Here's how the part is built. I have some questions about the finished solid (model axes, mm). Face numbers are marked on the shaded views. A direction names the side the tool comes from. Coordinates: 2 decimals unless noted, no trailing zeros. Write each loop counter-clockwise with the first axis right and the second up, starting at its lowest first coordinate (ties: lowest second). Pieces come first, ordered by that corner, then holes. Notation, with made-up numbers: (-13, 74) -> (16, 74) arc R17 cw to (16, 85) -> close; hole circle Ø3 at (21.5, -11). An arc over 180 degrees is marked (long way). Put each result on its own line as item: value. Start each with the question number.
Item 1: For pin 1 (12 mm diameter, centred on x = 14.5, y = 53, fed in from -Z); pin 2 (4 mm diameter, centred on y = 10, z = 292.5, fed in from +X); pin 3 (4 mm diameter, centred on x = 10, z = 116, fed in from +Y); pin 4 (5 mm diameter, centred on x = 20, z = 262.5, fed in from +Y), each with a flat end and sliding along its axis, tell me the tip position at first contact or that it passes through.
Item 2: I want a section at C-C, the plane x = 45. List the corners of the cut face in (y, z) for me.
Item 3: On a 3-axis mill with a long thin cutter (end or side, diameter ignored), from which of +Z, -Z, +X, -X, +Y, -Y can I reach the whole of each face in a straight line? I mean the marked faces 1 and 2. Say none if no direction works.
Item 4: I want a section at A-A, the plane z = 36. List the corners of the cut face in (x, y) for me.
Item 5: I need wall thicknesses on line 1 (X direction, y = 64, z = 130); line 2 (X direction, y = 4, z = 23). Which ranges of each line are inside material? Lowest first, please. Write a range as [from, to].
Item 6: I want a section at B-B, the plane y = 67.5. List the corners of the cut face in (x, z) for me, then the cut area to 3 significant figures.
Autodesk Inventor part; units mm, degrees
ref_plane "Start plane" through (0, 0, -10.521) normal (0, 0, 1) x (1, 0, 0)
ref_plane "End plane" through (0, 0, 342.7905) normal (0, 0, 1) x (1, 0, 0)
ref_plane "Work Plane3" through (50.8, 38.1, -10.521) normal (-0.3827, 0, -0.9239) x (-0.9239, 0, 0.3827)
ref_plane "Start plane" through (0, 0, -10.521) normal (0, 0, 1) x (1, 0, 0)
ref_plane "End plane" through (0, 0, 342.7905) normal (0, 0, 1) x (1, 0, 0)
sketch "Sketch" plane through (0, 0, 0) normal (0, 0, 1) x (1, 0, 0)
  line L0 (0, 76.2) -> (0, 0)
  line L1 (0, 0) -> (50.8, 0)
  line L2 (50.8, 0) -> (50.8, 2.7625)
  line L3 (48.8, 4.7625) -> (12.6365, 4.7625)
  line L4 (4.7625, 12.6365) -> (4.7625, 74.2)
  line L5 (2.7625, 76.2) -> (0, 76.2)
  line L6 (-7.0414, 0) -> (21.5385, 0) construction
  line L7 (0, -8.0414) -> (0, 34.5385) construction
  arc A0 (4.7625, 12.6365) -> (12.6365, 4.7625) centre (12.6365, 12.6365) ccw
  arc A1 (50.8, 2.7625) -> (48.8, 4.7625) centre (48.8, 2.7625) ccw
  arc A2 (4.7625, 74.2) -> (2.7625, 76.2) centre (2.7625, 74.2) ccw
  line L8 (0, 93.5453) -> (0, -24.9725) construction
  line L9 (-18.6925, 0) -> (62.8653, 0) construction
  point P0 (50.8, 4.7625)
  point P1 (4.7625, 4.7625)
  point P2 (4.7625, 76.2)
  dimension "d12" = 4.7625
  dimension "d13" = 76.2
  dimension "d14" = 50.8
  dimension "d15" = 0
  dimension "d16" = 4.7625
  dimension "d17" = 0
  dimension "d18" = 7.874
  dimension "d19" = 2
extrude "Body" add sketch "Sketch" along normal up to surface (353.3115 mm away) from surface at -10.521
sketch "Sketch3" plane through (0, 0, 0) normal (0, 0, 1) x (1, 0, 0)
  line L0 (0, 0) -> (10, 0)
ref_plane "Work Plane5" through (0, 0, 0) normal (0, -1, 0) x (1, 0, 0)
sketch "Sketch4" plane through (0, 0, 0) normal (0, -1, 0) x (1, 0, 0)
  line L0 (-2, -10.521) -> (12, -10.521)
  line L1 (-2, 342.7905) -> (12, 342.7905)
  dimension "d23" = 353.3115
ref_plane "Work Plane3" through (50.8, 38.1, -10.521) normal (-0.3827, 0, -0.9239) x (-0.9239, 0, 0.3827)
split "Split1" plane through (50.8, 38.1, -10.521) removes the side toward (-0.3827, 0, -0.9239)
ref_plane "Work Plane4" through (50.8, 38.1, 342.7905) normal (-0.3827, 0, 0.9239) x (0.9239, 0, 0.3827)
split "Split2" plane through (50.8, 38.1, 342.7905) removes the side toward (-0.3827, 0, 0.9239)
equation "\"d12\" = G_T"
equation "\"d13\" = G_H"
equation "\"d14\" = G_W"
equation "\"d16\" = G_T"
equation "\"d18\" = G_IR"
equation "\"d4\" = G_L"
equation "\"G_W\" = 50.8"
equation "\"G_H\" = 76.2"
equation "\"G_T\" = 4.7625"
equation "\"G_ER\" = 4.064"
equation "\"G_IR\" = 7.874"
equation "\"G_L\" = d23"
equation "\"ex\" = 0"
equation "\"ey\" = 0"
equation "\"G_OFFSET_START\" = 10.52102"
equation "\"G_OFFSET_END\" = 10.52102"
equation "\"d20\" = -G_OFFSET_START"
equation "\"d21\" = G_OFFSET_END + B_L"
equation "\"B_L\" = 332.26948"
properties part number "ANSI L 3 x 2 x 3_16 00000002"
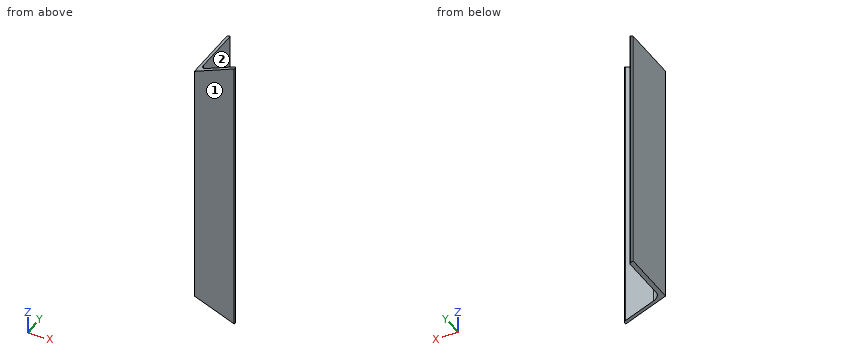
Calculated:
1. pin 1: passes through
1. pin 2: stops at x = 6.27
1. pin 3: stops at y = 6.27
1. pin 4: stops at y = 4.76
2. outline: (0, -8.12) -> (4.76, -8.12) -> (4.76, 340.39) -> (0, 340.39) -> close
3. face 1: +Z, -Z, +X, -X, -Y
3. face 2: +Z, -Z, +X, +Y
4. outline: (0, 0) -> (50.8, 0) -> (50.8, 2.76) arc R2 ccw to (48.8, 4.76) -> (12.64, 4.76) arc R7.87 cw to (4.76, 12.64) -> (4.76, 74.2) arc R2 ccw to (2.76, 76.2) -> (0, 76.2) -> close
5. line 1: x = [0, 4.76]
5. line 2: x = [0, 50.37]
6. outline: (0, 10.52) -> (4.76, 8.55) -> (4.76, 323.72) -> (0, 321.75) -> close
6. area: 1,490 mm2
